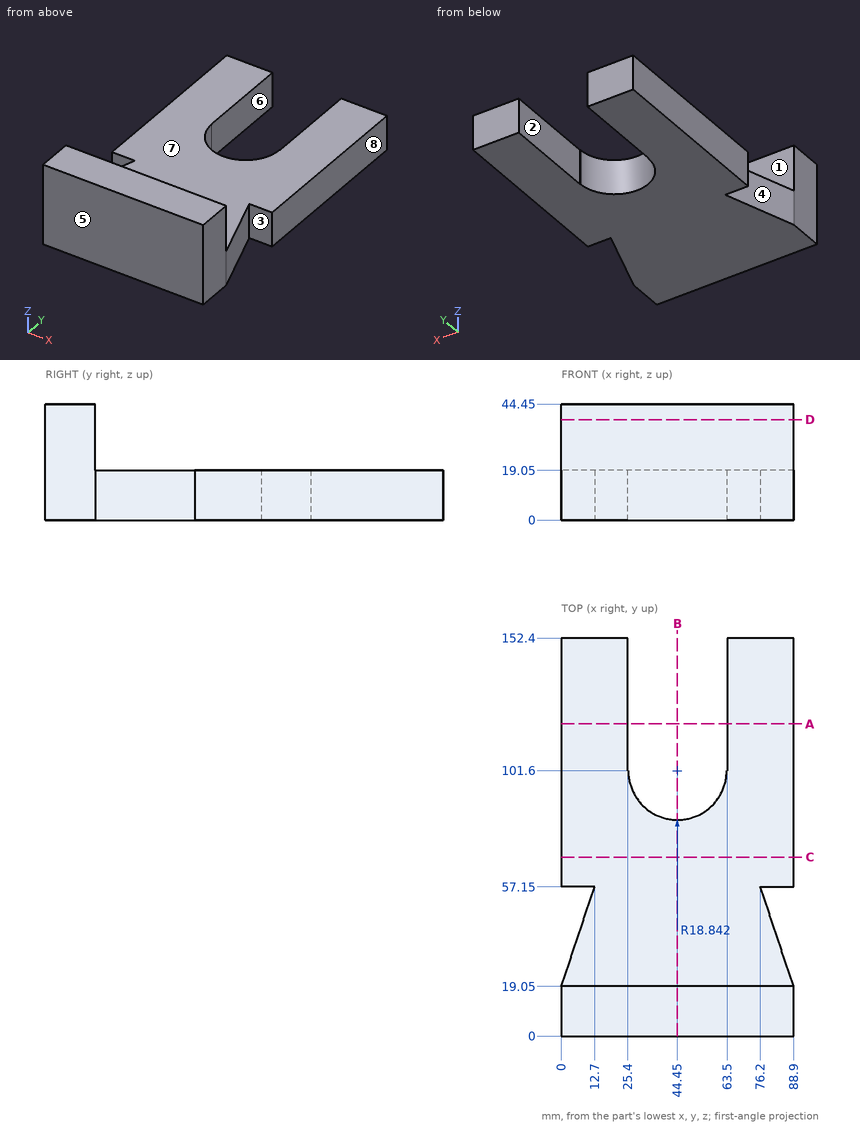
Geometry: see drawing. Coordinates: mm, zero at the bounding-box minimum. A direction names the side the tool comes from. Round coordinates to 2 decimals unless told otherwise and drop trailing zeros. Loops run counter-clockwise (first coordinate to the right, second up) from the corner with the lowest first, then second, coordinate; pieces in that order, holes last. Notation, with made-up numbers: (59, 42) - (82, 42) arc R28 ccw to (82, 81) - close; hole circle Ø2 at (70, 53.5). An arc over 180 degrees is marked (long way). Write item = value, one per line. Start each with the question number.
(1) Pin query (flat end, axial travel): pin 1 (6.5 mm diameter, centred on x = 83.5, z = 7, fed in from -Y); pin 2 (8 mm diameter, centred on x = 38.5, y = 87, fed in from +Z); pin 3 (4 mm diameter, centred on x = 64, z = 25, fed in from +Y). Return the tip coordinate at first contact, or that it passes through.
(2) Section query B-B, the plane x = 44.45. Output: boundary loops of the cut face in (y, z), plus the area to 3 significant figures.
(3) Pull-direction query (X, two-part tool) for the marked faces 6, 7 and 8; classes: +X half, -X half, draft (parallel to the pull), parting line (faces both ways), or undercut.
(4) Set-up query: the marked faces 1, 2, 3, 4 and 5. Return all of +Z, -Z, +X, -X, +Y, -Y with unobstructed straight access to the full face (end or side cutting, diameter ignored); none if empty.
(5) Section query C-C, the plane y = 68.5. Output: boundary loops of the cut face in (x, z).
(6) Ray query, line 1 along X through (y, z) = (107.5, 11.5); line 2 along Y through (x, z) = (10, 25.5). Return the intervals inside material, ascending. Write a range as from..to.
(7) Section query A-A, the plane y = 119.5. Output: boundary loops of the cut face in (x, z).
Conclusion:
q1.pin_1 = 0
q1.pin_2 = 19.05
q1.pin_3 = 19.05
q2.outline = (0, 0) - (82.76, 0) - (82.76, 19.05) - (19.05, 19.05) - (19.05, 44.45) - (0, 44.45) - close
q2.area = 2,060 mm2
q3.face_6 = undercut
q3.face_7 = draft
q3.face_8 = +X half
q4.face_1 = +Z, +X, -X, +Y
q4.face_2 = +Z, -Z, +Y
q4.face_3 = +Z, -Z, +X
q4.face_4 = +Z, -Z, -X
q4.face_5 = +Z, -Z, +X, -X, -Y
q5.outline = (0, 0) - (88.9, 0) - (88.9, 19.05) - (0, 19.05) - close
q6.line_1 = 0..25.4, 63.5..88.9
q6.line_2 = 0..19.05
q7.outline = (0, 0) - (25.4, 0) - (25.4, 19.05) - (0, 19.05) - close; (63.5, 0) - (88.9, 0) - (88.9, 19.05) - (63.5, 19.05) - close
